The model under review builds one solid part; all positions refer to its coordinate system, in mm. Round coordinates to 2 decimals unless told otherwise and drop trailing zeros. Write each loop counter-clockwise with the first axis right and the second up, starting at its lowest first coordinate (ties: lowest second). Pieces come first, ordered by that corner, then holes. Notation, with made-up numbers: (59, 54) - (117, 54) arc R21 cw to (117, 58) - close; hole circle Ø3 at (50.5, 8). An arc over 180 degrees is marked (long way). Return JSON: item names as keys, results as strings.
from build123d import *

# Parameters (mm, degrees)
F0_W     = 312.42
F0_H     = 327.66
F0_R     = 3.5687
F0_R_2   = 3.683
F0_R_3   = 2.1844
F1_DEPTH = 2.286
F2_W     = 6.35
F2_H     = 4.445
F2_W_2   = 5.08
F2_H_2   = 135.255
F2_H_3   = 144.145
F3_DEPTH = 2.287
F4_SIZE  = 13.97
F5_SIZE  = 6.35
F6_SIZE  = 3.175


with BuildPart() as f1:
    # F0 (on Top) → F1 (new body)
    with BuildSketch(Plane.XY):
        Rectangle(F0_W, F0_H)
        with Locations((-138.43, -151.13)):
            Circle(F0_R, mode=Mode.SUBTRACT)
        with Locations((-124.46, -130.81)):
            Circle(F0_R_2, mode=Mode.SUBTRACT)
        with Locations((-124.46, -116.84)):
            Circle(F0_R_3, mode=Mode.SUBTRACT)
        with Locations((-138.43, -96.52)):
            Circle(F0_R, mode=Mode.SUBTRACT)
        with Locations((-36.83, -151.13)):
            Circle(F0_R, mode=Mode.SUBTRACT)
        with Locations((-36.83, -96.52)):
            Circle(F0_R, mode=Mode.SUBTRACT)
        with Locations((-138.43, -6.985)):
            Circle(F0_R, mode=Mode.SUBTRACT)
        with Locations((-36.83, -6.985)):
            Circle(F0_R, mode=Mode.SUBTRACT)
        with Locations((2.54, -130.81)):
            Circle(F0_R_2, mode=Mode.SUBTRACT)
        with Locations((64.77, -151.13)):
            Circle(F0_R, mode=Mode.SUBTRACT)
        with Locations((2.54, -116.84)):
            Circle(F0_R_3, mode=Mode.SUBTRACT)
        with Locations((64.77, -96.52)):
            Circle(F0_R, mode=Mode.SUBTRACT)
        with Locations((105.41, -151.13)):
            Circle(F0_R, mode=Mode.SUBTRACT)
        with Locations((129.54, -130.81)):
            Circle(F0_R_2, mode=Mode.SUBTRACT)
        with Locations((105.41, -96.52)):
            Circle(F0_R, mode=Mode.SUBTRACT)
        with Locations((129.54, -116.84)):
            Circle(F0_R_3, mode=Mode.SUBTRACT)
        with Locations((64.77, -6.985)):
            Circle(F0_R, mode=Mode.SUBTRACT)
        with Locations((105.41, -6.985)):
            Circle(F0_R, mode=Mode.SUBTRACT)
        with Locations((146.05, -6.985)):
            Circle(F0_R, mode=Mode.SUBTRACT)
        with Locations((-124.46, 5.08)):
            Circle(F0_R_3, mode=Mode.SUBTRACT)
        with Locations((-124.46, 30.48)):
            Circle(F0_R_2, mode=Mode.SUBTRACT)
        with Locations((-124.46, 132.08)):
            Circle(F0_R_3, mode=Mode.SUBTRACT)
        with Locations((-138.43, 153.67)):
            Circle(F0_R, mode=Mode.SUBTRACT)
        with Locations((-124.46, 144.78)):
            Circle(F0_R_2, mode=Mode.SUBTRACT)
        with Locations((-36.83, 153.67)):
            Circle(F0_R, mode=Mode.SUBTRACT)
        with Locations((2.54, 5.08)):
            Circle(F0_R_3, mode=Mode.SUBTRACT)
        with Locations((2.54, 30.48)):
            Circle(F0_R_2, mode=Mode.SUBTRACT)
        with Locations((129.54, 5.08)):
            Circle(F0_R_3, mode=Mode.SUBTRACT)
        with Locations((129.54, 30.48)):
            Circle(F0_R_2, mode=Mode.SUBTRACT)
        with Locations((2.54, 132.08)):
            Circle(F0_R_3, mode=Mode.SUBTRACT)
        with Locations((2.54, 144.78)):
            Circle(F0_R_2, mode=Mode.SUBTRACT)
        with Locations((64.77, 153.67)):
            Circle(F0_R, mode=Mode.SUBTRACT)
        with Locations((105.41, 153.67)):
            Circle(F0_R, mode=Mode.SUBTRACT)
        with Locations((129.54, 132.08)):
            Circle(F0_R_3, mode=Mode.SUBTRACT)
        with Locations((129.54, 144.78)):
            Circle(F0_R_2, mode=Mode.SUBTRACT)
        with Locations((146.05, 153.67)):
            Circle(F0_R, mode=Mode.SUBTRACT)
    extrude(amount=F1_DEPTH)

    # F2 (on face) → F3 (cut, through all)
    with BuildSketch(Plane.XY.offset(2.286)):
        with BuildLine():
            ThreePointArc((-96.393, 159.385), (-93.218, 156.21), (-90.043, 159.385))
            Line((-90.043, 159.385), (-96.393, 159.385))
        make_face()
        with Locations((-93.218, 161.6075)):
            Rectangle(F2_W, F2_H)
        with Locations((-93.218, 166.0525)):
            Rectangle(F2_W, F2_H)
        with Locations((-27.178, 166.0525)):
            Rectangle(F2_W, F2_H)
        with Locations((-27.178, 161.6075)):
            Rectangle(F2_W, F2_H)
        with BuildLine():
            Line((-24.003, 159.385), (-30.353, 159.385))
            ThreePointArc((-30.353, 159.385), (-27.178, 156.21), (-24.003, 159.385))
        make_face()
        with Locations((21.082, 166.0525)):
            Rectangle(F2_W, F2_H)
        with Locations((21.082, 161.6075)):
            Rectangle(F2_W, F2_H)
        with BuildLine():
            Line((24.257, 159.385), (17.907, 159.385))
            ThreePointArc((17.907, 159.385), (21.082, 156.21), (24.257, 159.385))
        make_face()
        with Locations((78.232, 166.0525)):
            Rectangle(F2_W, F2_H)
        with Locations((78.232, 161.6075)):
            Rectangle(F2_W, F2_H)
        with BuildLine():
            Line((81.407, 159.385), (75.057, 159.385))
            ThreePointArc((75.057, 159.385), (78.232, 156.21), (81.407, 159.385))
        make_face()
        with Locations((135.382, 166.0525)):
            Rectangle(F2_W, F2_H)
        with Locations((135.382, 161.6075)):
            Rectangle(F2_W, F2_H)
        with BuildLine():
            Line((138.557, 159.385), (132.207, 159.385))
            ThreePointArc((132.207, 159.385), (135.382, 156.21), (138.557, 159.385))
        make_face()
        with Locations((153.67, 73.3425)):
            Rectangle(F2_W_2, F2_H_2)
        with Locations((153.67, -91.7575)):
            Rectangle(F2_W_2, F2_H_3)
    extrude(amount=-F3_DEPTH, mode=Mode.SUBTRACT)

    # F4
    f4_edges = [f1.edges().sort_by_distance(p)[0] for p in [
        (-156.21, 163.83, 1.143),
    ]]
    chamfer(f4_edges, length=F4_SIZE)

    # F5
    f5_edges = [f1.edges().sort_by_distance(p)[0] for p in [
        (-156.21, -163.83, 1.143),
        (151.13, -163.83, 1.143),
        (156.21, 163.83, 1.143),
    ]]
    chamfer(f5_edges, length=F5_SIZE)

    # F6
    f6_edges = [f1.edges().sort_by_distance(p)[0] for p in [
        (156.21, 140.97, 1.143),
        (156.21, 5.715, 1.143),
        (156.21, -19.685, 1.143),
    ]]
    chamfer(f6_edges, length=F6_SIZE)


solid = f1.part
(1) Clearance check with a flat-ended pin moving along its axis: pin 1 Ø0.7 at (y, z) = (161.5, 1.5) entering from +X. State where the tip first meets the part, or that it passes through.
Filled in:
{"pin 1": "stops at x = 152.54"}
(2) Add section B-B (y = 103). Write out the cut boundary in (x, z), plus the area to 3 significant figures.
Filled in:
{"outline": "(-156.21, 0) - (151.13, 0) - (151.13, 2.29) - (-156.21, 2.29) - close", "area": "703 mm2"}
(3) Wall thickness on line 1 (Y direction, x = -36.83, z = 1.8); line 2 (Y direction, x = 67.5, z = 2.1); line 3 (X direction, y = 93, z = 2.15): over which ranges is each line inside the solid? List them lowest first.
Filled in:
{"line 1": "y = -163.83 to -154.7, -147.56 to -100.09, -92.95 to -10.55, -3.42 to 150.1, 157.24 to 163.83", "line 2": "y = -163.83 to -153.43, -148.83 to -98.82, -94.22 to -9.28, -4.69 to 151.37, 155.97 to 163.83", "line 3": "x = -156.21 to 151.13"}
(4) Mouldability with a two-part tool opening along Y and no side actions: class faces 1 (the cylindrical face through (66.69, -93.51, 1.13)), 2 (the flat face through (-2, 2, 0)), 3 (the flat face through (-149.13, 156.94, 1.13)) as released by +Y, released by -Y, zero draft, split by the parting line, or undercut.
Filled in:
{"face 1": "undercut", "face 2": "zero draft", "face 3": "released by +Y"}
(5) Add section C-C (z = 1.8). Give the number of separate pieces and of enclosed holes in the cut face, plus the area to 3 significant figures.
Filled in:
{"separate pieces": "1", "enclosed holes": "36", "area": "99,300 mm2"}
(6) Add section A-A (y = -130.81). Write out the cut boundary in (x, z), plus the area to 3 significant figures.
Filled in:
{"outline": "(-156.21, 0) - (-128.14, 0) - (-128.14, 2.29) - (-156.21, 2.29) - close; (-120.78, 0) - (-1.14, 0) - (-1.14, 2.29) - (-120.78, 2.29) - close; (6.22, 0) - (125.86, 0) - (125.86, 2.29) - (6.22, 2.29) - close; (133.22, 0) - (151.13, 0) - (151.13, 2.29) - (133.22, 2.29) - close", "area": "652 mm2"}
